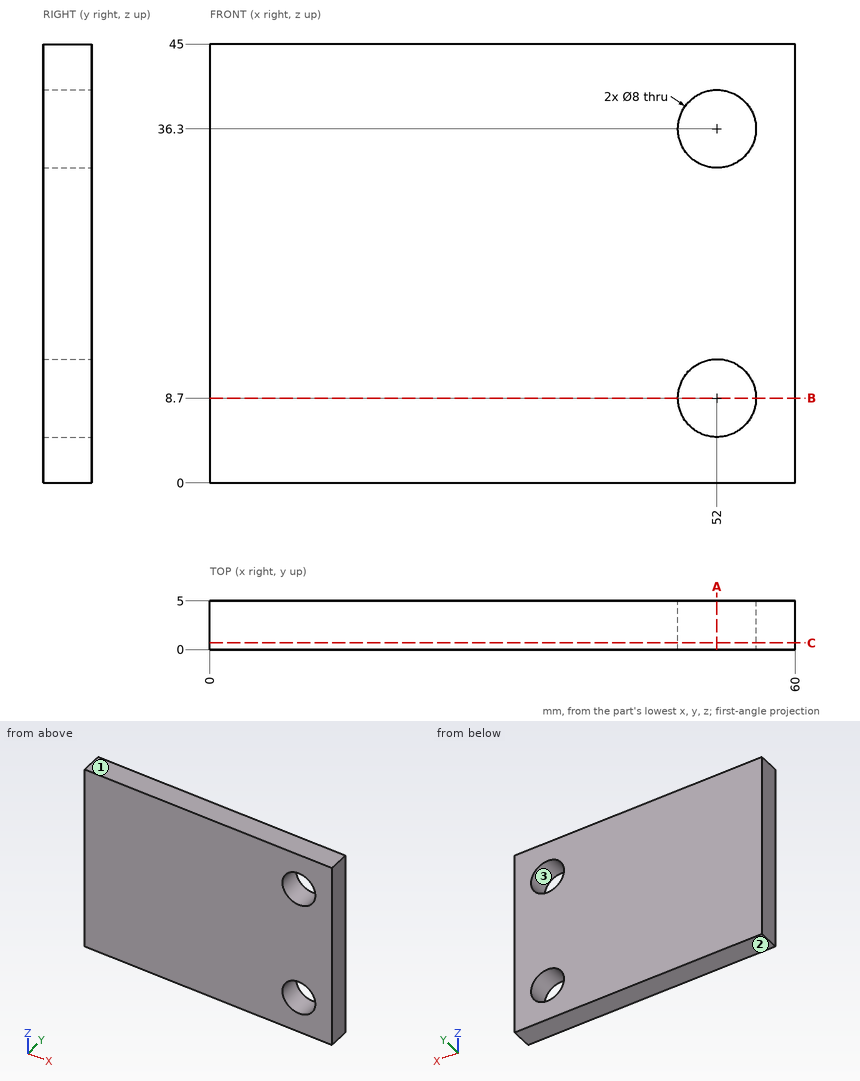
Here's the drawing with two shaded views (mm, measured from the low corner). I have some questions. Give positions to 0.01 mm unless a question says otherwise; leave off trailing zeros. Loops run counter-clockwise (first coordinate to the right, second up) from the corner with the lowest first, then second, coordinate; pieces in that order, holes last. Notation, with made-up numbers: M 77,21 L 136,21 A24 ccw 136,52 Z; hole C -10.5,8.25 d9. An arc over 180 degrees is marked long. One line per item, written item: value.
(1) We'd pull the mould along Z, two halves only. Please class the marked faces 1, 2 and 3: released by +Z, released by -Z, zero draft, split by the parting line, or undercut.
Returned:
face 1: released by +Z
face 2: released by -Z
face 3: undercut
(2) Suppose I cut it at A-A on x = 52. List the corners of the cut face in (y, z) for me.
Returned:
outline: M 0,0 L 5,0 L 5,4.7 L 0,4.7 Z; M 0,12.7 L 5,12.7 L 5,32.3 L 0,32.3 Z; M 0,40.3 L 5,40.3 L 5,45 L 0,45 Z
(3) Suppose I cut it at B-B on z = 8.7. List the corners of the cut face in (x, y) for me.
Returned:
outline: M 0,0 L 48,0 L 48,5 L 0,5 Z; M 56,0 L 60,0 L 60,5 L 56,5 Z
(4) I need wall thicknesses on line 1 (Z direction, x = 52, y = 1.4); line 2 (X direction, y = 2.8, z = 36.3); line 3 (Z direction, x = 48.5, y = 4.2). Which ranges of each line are inside material? Lowest first, please.
Returned:
line 1: 0 to 4.7, 12.7 to 32.3, 40.3 to 45
line 2: 0 to 48, 56 to 60
line 3: 0 to 6.76, 10.64 to 34.36, 38.24 to 45
(5) Will this pin go through, and if not, where does the flat tip stop? pin 1 (7 mm diameter, centred on x = 52, z = 8.7, fed in from -Y).
Returned:
pin 1: through
(6) Suppose I cut it at C-C on y = 0.7. List the corners of the cut face in (x, z) for me, plus the area to 3 significant figures.
Returned:
outline: M 0,0 L 60,0 L 60,45 L 0,45 Z; hole C 52,8.7 d8; hole C 52,36.3 d8
area: 2,600 mm^2
